```python
from build123d import *

# Parameters (mm, degrees)
F1_DEPTH = 38.1
F2_R     = 6.29457
F2_R_2   = 6.286061
F3_DEPTH = 82.296
F4_SIZE2 = 21.997045
F4_SIZE  = 38.1


with BuildPart() as f1:
    # F0 (on Front) → F1 (new body)
    with BuildSketch(Plane.XZ):
        Polygon((-62.048577, 25.4), (-62.048577, 0), (64.951423, 0), (64.951423, 25.4), (39.551423, 25.4), (26.851423, 50.8), (14.151423, 50.8), (14.151423, 50.661036), (-11.248577, 50.661036), (-11.248577, 50.8), (-23.948577, 50.8), (-36.648577, 25.4), align=None)
    extrude(amount=F1_DEPTH)

    # F2 (on Top) → F3 (cut)
    with BuildSketch(Plane.XY):
        with Locations((-49.085889, -18.490879)):
            Circle(F2_R)
        with Locations((53.66724, -19.472597)):
            Circle(F2_R_2)
    extrude(amount=F3_DEPTH, mode=Mode.SUBTRACT)

    # F4
    f4_edges = [f1.edges().sort_by_distance(p)[0] for p in [
        (1.451423, -38.1, 50.661036),
    ]]
    chamfer(f4_edges, length=F4_SIZE, length2=F4_SIZE2)


solid = f1.part
```
Can you work these out from the model? Positions are in its coordinate system, mm. A direction names the side the tool comes from. Give positions to 0.01 mm unless a question says otherwise; leave off trailing zeros. Order: outer loops, then holes, each group sorted by start corner. A loop starts at its lowest first (then second) coordinate and runs counter-clockwise, first axis right, second up. Notation, with made-up numbers: M 7.25,57 L 14.25,57 A18 ccw 14.25,68 Z; hole C 8.25,45.5 d6. An arc over 180 degrees is marked long. Write item = value, one per line. Start each with the question number.
Q1. Suppose I cut it at D-D (z = 36). Write out the boundary of the cut face in (x, y), plus the area to 3 significant figures.
Q2. Will these pins go through, and if not, where does the flat tip stop? pin 1 Ø20 at (x, y) = (53.67, -19.47) entering from -Z; pin 2 Ø5 at (x, y) = (4.5, -5.5) entering from +Z; pin 3 Ø3 at (y, z) = (-8.5, 42.5) entering from -X; pin 4 Ø10 at (y, z) = (-22, 31.5) entering from +X.
Q3. For faces 1 (the flat face through (-11.249, -32, 37)), 2 (the flat face through (21, -19, 50.8)), 3 (the flat face through (47, -19, 25.4)), 4 (the flat face through (2, -8, 50.661)), 5 (the flat face through (-44, -23, 25.4)), which set-ups out of +Z, -Z, +X, -X, +Y, -Y let a thin tool reach every point of the face, with its end or its side?
Q4. Suppose I cut it at A-A (x = -45.5). Write out the boundary of the cut face in (y, z).
Q5. Suppose I cut it at B-B (y = -22). Write out the boundary of the cut face in (x, z).
Q6. Suppose I cut it at C-C (x = -7). Write out the boundary of the cut face in (y, z).
Q7. I need wall thicknesses on probe 1 along X at (y, z) = (-14.5, 6.5); probe 2 along X at (y, z) = (-20.5, 11); probe 3 along Z at (x, y) = (42, -2.5). Which ranges of each line are inside material? Lowest first, please. Write a range as [from, to].
Check result:
q1.outline = M -31.35,-38.1 L -11.25,-38.1 L -11.25,-24.57 L 14.15,-24.57 L 14.15,-38.1 L 34.25,-38.1 L 34.25,0 L -31.35,0 Z
q1.area = 2,160 mm2
q2.pin_1 = 0
q2.pin_2 = 50.66
q2.pin_3 = -28.85
q2.pin_4 = 39
q3.face_1 = +Z, -Y
q3.face_2 = +Z, +X, -X, +Y, -Y
q3.face_3 = +Z, +X, +Y, -Y
q3.face_4 = +Z, +Y, -Y
q3.face_5 = +Z, -X, +Y, -Y
q4.outline = M -38.1,0 L -23.66,0 L -23.66,25.4 L -38.1,25.4 Z; M -13.32,0 L 0,0 L 0,25.4 L -13.32,25.4 Z
q5.outline = M -62.05,0 L -54.31,0 L -54.31,25.4 L -62.05,25.4 Z; M -43.86,0 L 47.91,0 L 47.91,25.4 L 39.55,25.4 L 26.85,50.8 L 14.15,50.8 L 14.15,40.45 L -11.25,40.45 L -11.25,50.8 L -23.95,50.8 L -36.65,25.4 L -43.86,25.4 Z; M 59.42,0 L 64.95,0 L 64.95,25.4 L 59.42,25.4 Z
q6.outline = M -38.1,0 L 0,0 L 0,50.66 L -16.1,50.66 L -38.1,12.56 Z
q7.probe_1 = [-62.05, -53.95], [-44.22, 49.82], [57.51, 64.95]
q7.probe_2 = [-62.05, -55.05], [-43.12, 47.47], [59.87, 64.95]
q7.probe_3 = [0, 25.4]
